```python
from build123d import *

# Parameters (mm, degrees)
SKETCH1_R            = 7.5
BOSS_EXTRUDE1_DEPTH  = 10
SKETCH2_R            = 35
SKETCH2_R_2          = 30
BOSS_EXTRUDE2_DEPTH  = 48
BOSS_EXTRUDE3_DEPTH  = 6
BOSS_EXTRUDE6_DEPTH  = 3
RIB3_REACH           = 161.7
SKETCH5_WALLS_W      = 6
SKETCH5_WALLS_H      = 381.399436442
FILLET1_R            = 16
SKETCH6_R            = 14
SKETCH6_R_2          = 6
BOSS_EXTRUDE7_DEPTH  = 32.5
BOSS_EXTRUDE8_DEPTH  = 32.5
BOSS_EXTRUDE9_REACH  = 152.18
SKETCH8_W            = 14.472243623
SKETCH8_H            = 28
BOSS_EXTRUDE10_REACH = 152.18
SKETCH9_W            = 14.472243623
SKETCH9_H            = 28
SKETCH10_W           = 3
SKETCH10_H           = 122.594000843
CUT_EXTRUDE1_DEPTH   = 32.5


with BuildPart() as part:
    # Sketch1 → Boss-Extrude1 (new body)
    with BuildSketch(Plane(origin=(0, 0, 0), x_dir=(1, 0, 0), z_dir=(0, 1, 0))):
        with BuildLine():
            Line((-54, 21), (54, 21))
            ThreePointArc((54, 21), (58.242640687, 19.242640687), (60, 15))
            Line((60, 15), (60, -15))
            ThreePointArc((60, -15), (58.242640687, -19.242640687), (54, -21))
            Line((54, -21), (-54, -21))
            ThreePointArc((-54, -21), (-58.242640687, -19.242640687), (-60, -15))
            Line((-60, -15), (-60, 15))
            ThreePointArc((-60, 15), (-58.242640687, 19.242640687), (-54, 21))
        make_face()
        with Locations(Location((-45, 0, 0), (0, 0, 270))):
            Circle(SKETCH1_R, mode=Mode.SUBTRACT)
        with Locations(Location((45, 0, 0), (0, 0, 270))):
            Circle(SKETCH1_R, mode=Mode.SUBTRACT)
    extrude(amount=BOSS_EXTRUDE1_DEPTH)



with BuildPart() as body_2:
    # Sketch2 → Boss-Extrude2 (new body)
    with BuildSketch(Plane.XY.offset(21)):
        with Locations((0, 105)):
            Circle(SKETCH2_R)
        with Locations((0, 105)):
            Circle(SKETCH2_R_2, mode=Mode.SUBTRACT)
    extrude(amount=-BOSS_EXTRUDE2_DEPTH)


with BuildPart() as part_1:
    add(part.part)

    add(body_2.part)  # Boss-Extrude3 merges body 2
    # Sketch3 → Boss-Extrude3 (add)
    with BuildSketch(Plane(origin=(0, 0, -21), x_dir=(-1, 0, 0), z_dir=(0, 0, -1))):
        with BuildLine():
            Line((-35, 10), (35, 10))
            Line((35, 10), (35, 105))
            ThreePointArc((35, 105), (0, 70), (-35, 105))
            Line((-35, 105), (-35, 10))
        make_face()
    extrude(amount=-BOSS_EXTRUDE3_DEPTH)

    # Sketch4 → Boss-Extrude6 (add, symmetric)
    with BuildSketch(Plane(origin=(0, 0, 0), x_dir=(0, 0, -1), z_dir=(1, 0, 0))):
        Polygon((27, 70), (21, 20), (21, 70), (21, 73), (27, 73), align=None)
    extrude(amount=BOSS_EXTRUDE6_DEPTH, both=True)

    # Sketch5 walls → Rib3 (add, up to next)
    with BuildSketch(Plane.XY.offset(21), mode=Mode.PRIVATE) as rib3_sk1:
        with Locations((0, 40)):
            Rectangle(SKETCH5_WALLS_W, SKETCH5_WALLS_H)
    rib3_tool1 = extrude(rib3_sk1.sketch, amount=-RIB3_REACH, mode=Mode.PRIVATE) - part_1.part
    add(rib3_tool1.solids().sort_by_distance((0, 40, 21))[0])

    # Fillet1
    fillet1_edges = [part_1.edges().sort_by_distance(p)[0] for p in [
        (-35, 10, -18),
        (35, 10, -18),
    ]]
    fillet(fillet1_edges, radius=FILLET1_R)



with BuildPart() as body_2_2:
    # Sketch6 → Boss-Extrude7 (new, symmetric)
    with BuildSketch(Plane(origin=(0, 0, 0), x_dir=(0, 0, -1), z_dir=(1, 0, 0))):
        with Locations((7, 198.776584802)):
            Circle(SKETCH6_R)
        with Locations((7, 198.776584802)):
            Circle(SKETCH6_R_2, mode=Mode.SUBTRACT)
    extrude(amount=BOSS_EXTRUDE7_DEPTH, both=True)


with BuildPart() as part_2:
    add(part_1.part)

    add(body_2_2.part)  # Boss-Extrude8 merges body 2 2
    # Sketch7 → Boss-Extrude8 (add, symmetric)
    with BuildSketch(Plane(origin=(0, 0, 0), x_dir=(0, 0, -1), z_dir=(1, 0, 0))):
        with BuildLine():
            Line((21, 198.776584802), (21, 140))
            Line((21, 140), (21, 135))
            Line((21, 135), (-7, 135))
            Line((-7, 135), (-7, 140))
            Line((-7, 140), (-7, 198.776584802))
            ThreePointArc((-7, 198.776584802), (7, 184.776584802), (21, 198.776584802))
        make_face()
    extrude(amount=BOSS_EXTRUDE8_DEPTH, both=True)

    # Sketch8 → Boss-Extrude9 (add, up to next)
    with BuildSketch(Plane.XZ.offset(-135), mode=Mode.PRIVATE) as boss_extrude9_sk1:
        with Locations((25.263878189, -7)):
            Rectangle(SKETCH8_W, SKETCH8_H)
    boss_extrude9_tool1 = extrude(boss_extrude9_sk1.sketch, amount=BOSS_EXTRUDE9_REACH, mode=Mode.PRIVATE) - part_2.part
    add(boss_extrude9_tool1.solids().sort_by_distance((25.263878, 135, -7))[0])

    # Sketch9 → Boss-Extrude10 (add, up to next)
    with BuildSketch(Plane.XZ.offset(-135), mode=Mode.PRIVATE) as boss_extrude10_sk1:
        with Locations((-25.263878189, -7)):
            Rectangle(SKETCH9_W, SKETCH9_H)
    boss_extrude10_tool1 = extrude(boss_extrude10_sk1.sketch, amount=BOSS_EXTRUDE10_REACH, mode=Mode.PRIVATE) - part_2.part
    add(boss_extrude10_tool1.solids().sort_by_distance((-25.263878, 135, -7))[0])

    # Sketch10 → Cut-Extrude1 (cut, symmetric)
    with BuildSketch(Plane.XY):
        with Locations((0, 170.584475275)):
            Rectangle(SKETCH10_W, SKETCH10_H)
    extrude(amount=CUT_EXTRUDE1_DEPTH, both=True, mode=Mode.SUBTRACT)


solid = part_2.part
```
Input: part model. Units: mm. Frame: model coordinates. A direction names the side the tool comes from. Coordinates: 2 decimals unless noted, no trailing zeros. Write each loop counter-clockwise with the first axis right and the second up, starting at its lowest first coordinate (ties: lowest second). Pieces come first, ordered by that corner, then holes. Notation, with made-up numbers: (-18.75, 4.25) - (37.25, 4.25) arc R20 ccw to (37.25, 33.25) - close; hole circle Ø7 at (24, 5). An arc over 180 degrees is marked (long way). Put each result on its own line as item: value. Start each with the question number.
1) Contact query for flat-ended pins moving along their axis: pin 1 (5 mm diameter, centred on x = 28.5, z = 14.5, fed in from +Y); pin 2 (6.5 mm diameter, centred on y = 60, z = -18.5, fed in from -X); pin 3 (14.5 mm diameter, centred on x = 29, y = 38.5, fed in from +Z); pin 4 (12 mm diameter, centred on x = 45, z = 0, fed in from +Y). Output: stop coordinate, or through.
2) Cut plane A-A (x = -12). Return the cut outline in (y, z), plus the area to 3 significant figures.
3) Ray query, L1, parallel to X at y = 6, z = 0; L2, parallel to X at y = 105, z = 1; L3, parallel to Y at x = 13, z = 18. Return the intervals inside material, ascending.
4) Reachability of faces 4 (the face through (-1.5, 165, -8)), 5 (the face through (3, 51, -23)), 6 (the face through (32.5, 166, -7)) from +Z, -Z, +X, -X, +Y, -Y: full face, straight path, thin tool, end or side. Return the list, or none.
5) Cut plane B-B (y = 43). Return the cut outline in (x, z).
6) Mould query, pull axis Y, two halves, no side actions, for faces 1 (the face through (33.06, 93.51, -2.66)), 2 (the face through (1, 0, 0)), 3 (the face through (-58.289, 4.93, -19.196)). Classes: pulls with the +Y half, pulls with the -Y half, needs draft (parallel to the pull), parting line crosses it, or undercut.
7) Cut plane D-D (x = 49). Return the cut outline in (y, z), plus the area to 3 significant figures.
8) Cut plane C-C (z = 5). Return the cut outline in (x, y), plus the area to 3 significant figures.
Resolved:
1. pin 1: stops at y = 128.43
1. pin 2: stops at x = -35
1. pin 3: stops at z = -15
1. pin 4: passes through
2. outline: (0, -21) - (72.12, -21) - (72.12, -27) - (77.5, -27) - (77.5, 21) - (72.12, 21) - (72.12, -15) - (10, -15) - (10, 21) - (0, 21) - close; (132.5, -27) - (137.88, -27) - (137.88, -21) - (198.78, -21) arc R14 ccw to (198.78, 7) - (137.88, 7) - (137.88, 21) - (132.5, 21) - close; hole circle Ø12 at (198.78, -7)
2. area: 3,210 mm2
3. L1: x = -60 to -52.5, -37.5 to 37.5, 52.5 to 60
3. L2: x = -35 to -30, 30 to 35
3. L3: y = 0 to 10, 72.5 to 77.96, 132.04 to 137.5
4. face 4: +Z, -Z, +Y
4. face 5: -Z, +X, -Y
4. face 6: +Z, -Z, +X, +Y
5. outline: (-35, -21) - (-3, -21) - (-3, -23.76) - (3, -23.76) - (3, -21) - (35, -21) - (35, -15) - (3, -15) - (3, 21) - (-3, 21) - (-3, -15) - (-35, -15) - close
6. face 1: undercut
6. face 2: pulls with the -Y half
6. face 3: needs draft
7. outline: (0, -21) - (10.13, -21) - (10.13, -15) - (10, -15) - (10, -6.34) - (0, -6.34) - close; (0, 6.34) - (10, 6.34) - (10, 21) - (0, 21) - close
7. area: 294 mm2
8. outline: (-60, 0) - (-50.59, 0) - (-50.59, 10) - (-60, 10) - close; (-39.41, 0) - (39.41, 0) - (39.41, 10) - (3, 10) - (3, 70.13) arc R35 ccw to (32.5, 117.99) - (32.5, 205.99) - (1.5, 205.99) - (1.5, 134.96) arc R30 cw (long way) to (-1.5, 134.96) - (-1.5, 205.99) - (-32.5, 205.99) - (-32.5, 117.99) arc R35 ccw to (-3, 70.13) - (-3, 10) - (-39.41, 10) - close; (50.59, 0) - (60, 0) - (60, 10) - (50.59, 10) - close
8. area: 6,830 mm2
